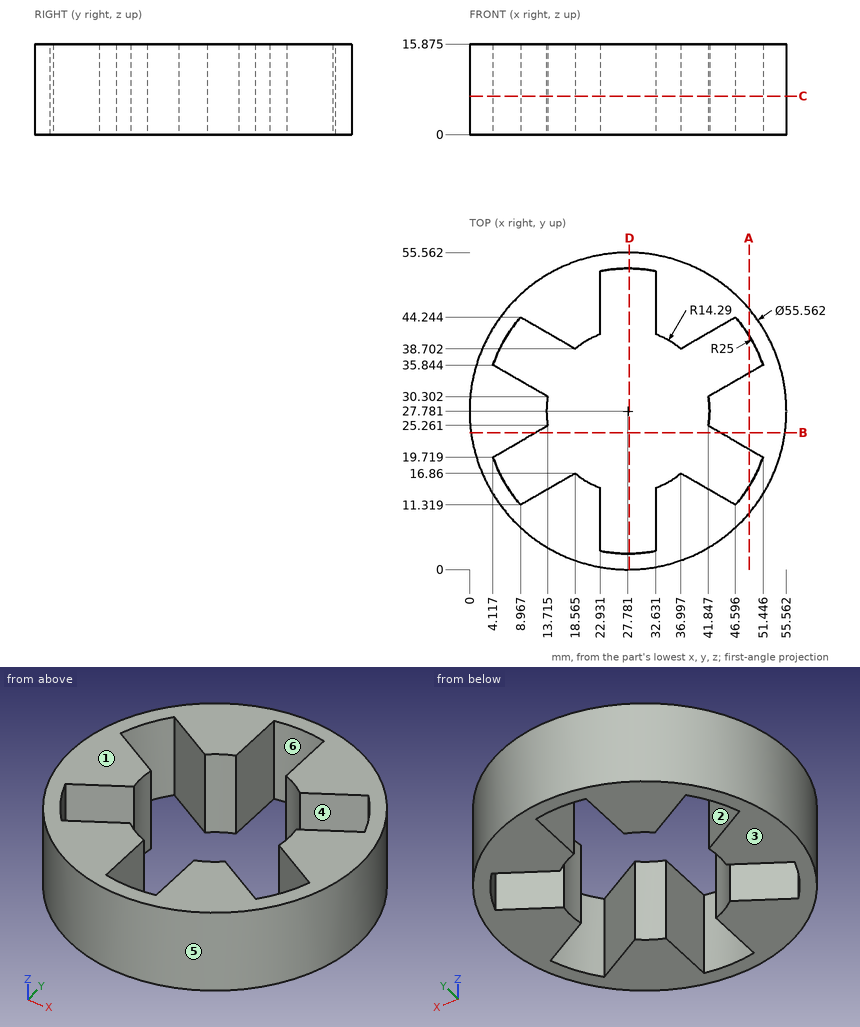
Answer from the drawing. Dimensions are ordinates in mm from the lowest x, y and z of the part. A direction names the side the tool comes from. Round coordinates to 2 decimals unless told otherwise and drop trailing zeros. Write each loop counter-clockwise with the first axis right and the second up, starting at its lowest first coordinate (ties: lowest second). Pieces come first, ordered by that corner, then holes.
1. Which of the six approach directions +Z, -Z, +X, -X, +Y, -Y give full straight-line access (tool end or side, diameter ignored) to the marked faces 1 and 2?
2. The part is cut by section A-A, the plane x = 49. State how many separate pieces and enclosed holes the cut face has, then the cut area to 3 significant figures.
3. Straight lines are drawn through the part: L1, parallel to Y at x = 11.5, z = 5.25; L2, parallel to Y at x = 32, z = 2.5; L3, parallel to Y at x = 47, z = 11.25 (1 decimal). For each, find the intervals that lie inside material, in ascending order.
4. Determine the mould class of the marked faces 3, 4, 5 and 6 for opening direction X: pulls with the +X half, pulls with the -X half, needs draft (parallel to the pull), parting line crosses it, or undercut.
5. The part is cut by section B-B, the plane y = 24. Determine the outline of the cut face in (x, z) (1 decimal), then the cut area to 3 significant figures.
6. The part is cut by section C-C, the plane z = 6.75. Determine the outline of the cut face in (x, y) (1 decimal), then the cut area to 3 significant figures.
7. The part is cut by section D-D, the plane x = 28. Determine the outline of the cut face in (y, z) (1 decimal).
8. Given pin 1 Ø6 at (y, z) = (12.5, 7.5) entering from -X; pin 2 Ø4 at (y, z) = (19, 14) entering from +X; pin 3 Ø2 at (y, z) = (21.5, 8) entering from +X; pin 4 Ø4 at (y, z) = (26.5, 3.5) entering from -X, each flat-ended and moving along its own axis, determine where each tip first touches the part or whether it passes through.
Values:
1. face 1: +Z, +X, -X, +Y, -Y
1. face 2: +Z, -Z
2. separate pieces: 3
2. enclosed holes: 0
2. area: 361 mm2
3. L1: y = 5.27 to 12.78, 23.98 to 31.58, 42.78 to 50.29
3. L2: y = 0.32 to 3.14, 52.42 to 55.24
3. L3: y = 7.7 to 11.8, 22.3 to 33.3, 43.8 to 47.8
4. face 3: needs draft
4. face 4: undercut
4. face 5: parting line crosses it
4. face 6: undercut
5. outline: (0.3, 0) - (11.5, 0) - (11.5, 15.9) - (0.3, 15.9) - close; (44, 0) - (55.3, 0) - (55.3, 15.9) - (44, 15.9) - close
5. area: 358 mm2
6. outline: circle Ø55.6 at (27.8, 27.8); hole (4.1, 19.7) arc R25 ccw to (9, 11.3) - (18.6, 16.9) arc R14.3 ccw to (22.9, 14.3) - (22.9, 3.3) arc R25 ccw to (32.6, 3.3) - (32.6, 14.3) arc R14.3 ccw to (37, 16.9) - (46.6, 11.3) arc R25 ccw to (51.4, 19.7) - (41.8, 25.3) arc R14.3 ccw to (41.8, 30.3) - (51.4, 35.8) arc R25 ccw to (46.6, 44.2) - (37, 38.7) arc R14.3 ccw to (32.6, 41.2) - (32.6, 52.3) arc R25 ccw to (22.9, 52.3) - (22.9, 41.2) arc R14.3 ccw to (18.6, 38.7) - (9, 44.2) arc R25 ccw to (4.1, 35.8) - (13.7, 30.3) arc R14.3 ccw to (13.7, 25.3) - close
6. area: 1,150 mm2
7. outline: (0, 0) - (2.8, 0) - (2.8, 15.9) - (0, 15.9) - close; (52.8, 0) - (55.6, 0) - (55.6, 15.9) - (52.8, 15.9) - close
8. pin 1: stops at x = 2.86
8. pin 2: stops at x = 54.72
8. pin 3: stops at x = 55.06
8. pin 4: stops at x = 0
